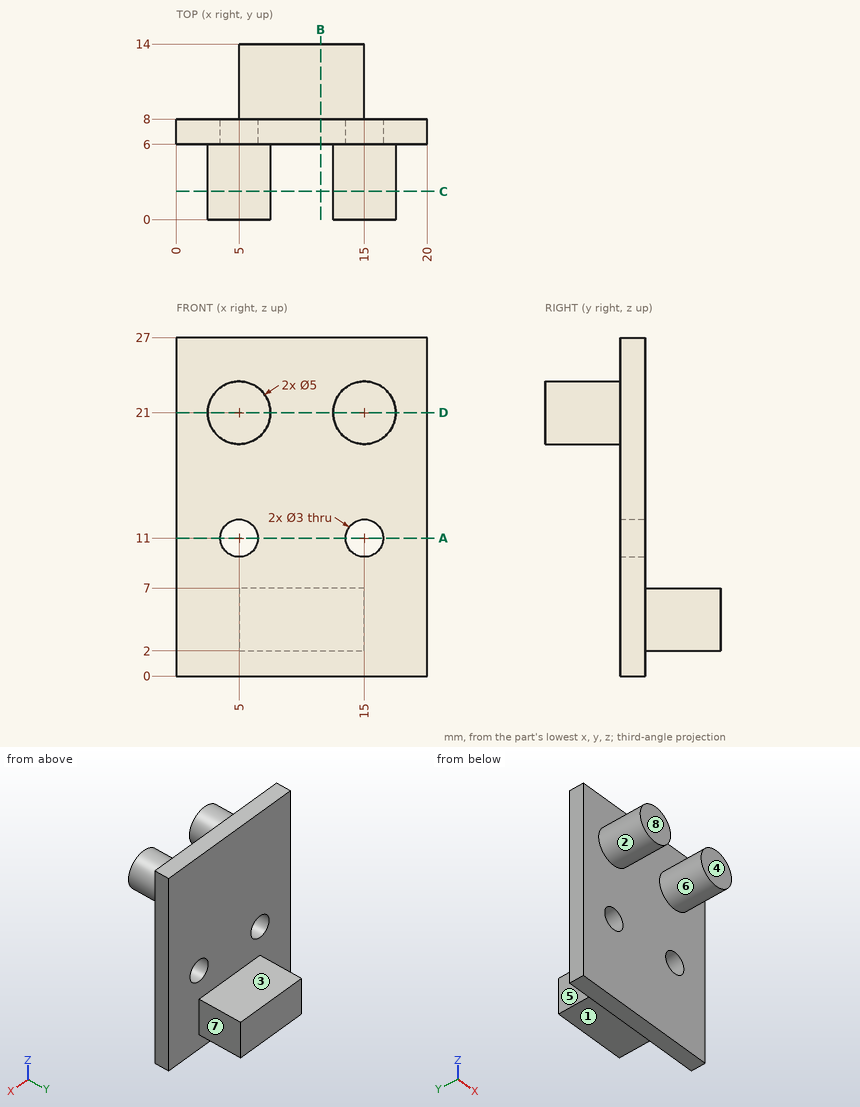
Could you check a few things on this drawing? It's one solid part, dimensions in mm from its lowest x, y, z. A direction names the side the tool comes from. Give positions to 0.01 mm unless a question says otherwise; leave off trailing zeros. Order: outer loops, then holes, each group sorted by start corner. A loop starts at its lowest first (then second) coordinate and runs counter-clockwise, first axis right, second up.
1. Suppose I cut it at B-B (x = 11.5). Write out the boundary of the cut face in (y, z).
Answers below:
outline: (6, 0) - (8, 0) - (8, 2) - (14, 2) - (14, 7) - (8, 7) - (8, 27) - (6, 27) - close
2. Which directions (+Z, -Z, +X, -X, +Y, -Y) give clear straight access to the entire face, cutting with the end or side of a thin tool? Please do the marked faces 1, 2, 3 and 4.
Answers below:
face 1: -Z, +X, -X, +Y
face 2: -Y
face 3: +Z, +X, -X, +Y
face 4: +Z, -Z, +X, -X, -Y
3. For pin 1 (1 mm diameter, centred on x = 15, y = 10, fed in from -Z); pin 2 (3 mm diameter, centred on x = 11, y = 11, fed in from +Z); pin 3 (3.5 mm diameter, centred on x = 15, z = 11, fed in from -Y), each with a flat end and sliding along its axis, tell me the tip position at first contact or that it passes through.
Answers below:
pin 1: stops at z = 2
pin 2: stops at z = 7
pin 3: stops at y = 6
4. Suppose I cut it at D-D (z = 21). Write out the boundary of the cut face in (x, y), plus the area to 3 significant figures.
Answers below:
outline: (0, 6) - (2.5, 6) - (2.5, 0) - (7.5, 0) - (7.5, 6) - (12.5, 6) - (12.5, 0) - (17.5, 0) - (17.5, 6) - (20, 6) - (20, 8) - (0, 8) - close
area: 100 mm2
5. Thinking about a two-plate mould opening in X: for the marked faces 5, 6, 7 and 8, which applies, +X half, -X half, draft (parallel to the pull), parting line (faces both ways), or undercut?
Answers below:
face 5: -X half
face 6: undercut
face 7: +X half
face 8: draft
6. I need wall thicknesses on L1, parallel to X at y = 7.45, z = 11; L2, parallel to Z at x = 15, y = 6.45; L3, parallel to Y at x = 4.75, z = 9. Which ranges of each line are inside material? Lowest first, please.
Answers below:
L1: x = 0 to 3.5, 6.5 to 13.5, 16.5 to 20
L2: z = 0 to 9.5, 12.5 to 27
L3: y = 6 to 8
7. Suppose I cut it at A-A (z = 11). Write out the boundary of the cut face in (x, y), plus the area to 3 significant figures.
Answers below:
outline: (0, 6) - (3.5, 6) - (3.5, 8) - (0, 8) - close; (6.5, 6) - (13.5, 6) - (13.5, 8) - (6.5, 8) - close; (16.5, 6) - (20, 6) - (20, 8) - (16.5, 8) - close
area: 28.0 mm2
8. Suppose I cut it at C-C (y = 2.25). Write out the boundary of the cut face in (x, z).
Answers below:
outline: circle Ø5 at (5, 21); circle Ø5 at (15, 21)
